from build123d import *

# Parameters (mm, degrees)
RESSALTO_EXTRUS_O1_DEPTH  = 5.25
CORTE_EXTRUS_O2_DEPTH     = 3.55
ESBO_O8_R                 = 1
CORTE_EXTRUS_O5_DEPTH     = 1.55
ESBO_O6_W                 = 1.275
ESBO_O6_H                 = 0.25
RESSALTO_EXTRUS_O2_DEPTH  = 0.025
ESBO_O7_W                 = 1.275
ESBO_O7_H                 = 0.25
CORTE_EXTRUS_O6_START     = -0.25
CORTE_EXTRUS_O6_DEPTH     = 0.25
ESBO_O10_W                = 0.445
ESBO_O10_H                = 0.25
RESSALTO_EXTRUS_O3_DEPTH  = 3.4
SIMETR_A1_COPY_1_SKETCH_W = 1.275
SIMETR_A1_COPY_1_SKETCH_H = 0.25
SIMETR_A1_COPY_1_DEPTH    = 0.025
SIMETR_A1_COPY_2_SKETCH_W = 1.275
SIMETR_A1_COPY_2_SKETCH_H = 0.25
SIMETR_A1_START           = -0.25
SIMETR_A1_COPY_3_DEPTH    = 0.25
SIMETR_A1_COPY_4_SKETCH_W = 0.445
SIMETR_A1_COPY_4_SKETCH_H = 0.25
SIMETR_A1_COPY_4_DEPTH    = 3.4


with BuildPart() as part:
    # Esboço1 → Ressalto-extrusão1 (new, symmetric)
    with BuildSketch(Plane(origin=(0, 0, 0), x_dir=(0, 0, -1), z_dir=(1, 0, 0))):
        Polygon((0.9, 3.1), (0.9, -3.1), (2.45, -3.3), (4, -3.1), (4, 3.1), (2.45, 3.3), align=None)
    extrude(amount=RESSALTO_EXTRUS_O1_DEPTH, both=True)

    # Esboço3 → Corte-extrusão2 (cut, symmetric)
    with BuildSketch(Plane(origin=(0, 0, 0), x_dir=(1, 0, 0), z_dir=(0, 1, 0))):
        Polygon((-5.25, 2.45), (-5.019897634, 4.376835982), (-6.186348907, 4.376835982), (-6.186348907, 0.523164018), (-5.019897634, 0.523164018), align=None)
    corte_extrus_o2 = extrude(amount=CORTE_EXTRUS_O2_DEPTH, both=True, mode=Mode.SUBTRACT)

    # Espelhar1: Corte-extrusão2 across plane
    add(corte_extrus_o2.mirror(Plane(origin=(0, 0, 0), x_dir=(0, 0, 1), z_dir=(1, 0, 0))), mode=Mode.SUBTRACT)

    # Esboço8 → Corte-extrusão5 (cut)
    with BuildSketch(Plane(origin=(0, 0, -4), x_dir=(-1, 0, 0), z_dir=(0, 0, -1))):
        with Locations((5.064899312, 0)):
            Circle(ESBO_O8_R)
    extrude(amount=-CORTE_EXTRUS_O5_DEPTH, mode=Mode.SUBTRACT)

    # Esboço6 → Ressalto-extrusão2 (add, symmetric)
    with BuildSketch(Plane(origin=(0, 3.3, 0), x_dir=(1, 0, 0), z_dir=(0, 1, 0))):
        with Locations((-3.8, 2.45)):
            Rectangle(ESBO_O6_W, ESBO_O6_H)
    ressalto_extrus_o2 = extrude(amount=RESSALTO_EXTRUS_O2_DEPTH, both=True)

    # Varredura1: sweep along a curve in space
    with BuildLine() as varredura1_path:
        Line((-3.8, 3.325, -2.45), (-3.8, 3.51, -2.45))
        ThreePointArc((-3.8, 3.51, -2.45), (-3.8, 3.722132034, -2.362132034), (-3.8, 3.81, -2.15))
        Line((-3.8, 3.81, -2.15), (-3.8, 3.81, 0.35))
    # Esboço7 → Varredura1 (sweep)
    with BuildSketch(Plane(origin=(0, 3.325, 0), x_dir=(1, 0, 0), z_dir=(0, 1, 0))):
        with Locations((-3.8, 2.45)):
            Rectangle(ESBO_O7_W, ESBO_O7_H)
    varredura1 = sweep(path=varredura1_path.line)

    # Esboço9 → Corte-extrusão6 (cut)
    with BuildSketch(Plane(origin=(0, 3.935, 0), x_dir=(1, 0, 0), z_dir=(0, 1, 0)).offset(CORTE_EXTRUS_O6_START)):
        Polygon((-4.0225, -0.35), (-4.4375, 0.55), (-4.4375, -0.55), (-3.1625, -0.55), (-3.1625, 0.55), (-3.5775, -0.35), align=None)
    corte_extrus_o6 = extrude(amount=CORTE_EXTRUS_O6_DEPTH, mode=Mode.SUBTRACT)

    # Esboço10 → Ressalto-extrusão3 (add)
    with BuildSketch(Plane.XY.offset(0.35)):
        with Locations((-3.8, 3.81)):
            Rectangle(ESBO_O10_W, ESBO_O10_H)
    ressalto_extrus_o3 = extrude(amount=RESSALTO_EXTRUS_O3_DEPTH)

    # Espelhar2: Ressalto-extrusão2, Varredura1, Corte-extrusão6, Ressalto-extrusão3 across plane
    add(ressalto_extrus_o2.mirror(Plane.ZX))
    add(varredura1.mirror(Plane.ZX))
    add(corte_extrus_o6.mirror(Plane.ZX), mode=Mode.SUBTRACT)
    add(ressalto_extrus_o3.mirror(Plane.ZX))

    # Simetría1: Ressalto-extrusão2, Varredura1, Corte-extrusão6, Ressalto-extrusão3 across plane
    add(ressalto_extrus_o2.mirror(Plane(origin=(0, 0, 0), x_dir=(0, 0, 1), z_dir=(1, 0, 0))))
    add(varredura1.mirror(Plane(origin=(0, 0, 0), x_dir=(0, 0, 1), z_dir=(1, 0, 0))))
    add(corte_extrus_o6.mirror(Plane(origin=(0, 0, 0), x_dir=(0, 0, 1), z_dir=(1, 0, 0))), mode=Mode.SUBTRACT)
    add(ressalto_extrus_o3.mirror(Plane(origin=(0, 0, 0), x_dir=(0, 0, 1), z_dir=(1, 0, 0))))

    # Simetría1 copy 1 sketch → Simetría1 copy 1 (add, symmetric)
    with BuildSketch(Plane(origin=(0, -3.3, 0), x_dir=(-1, 0, 0), z_dir=(0, -1, 0))):
        with Locations((-3.8, 2.45)):
            Rectangle(SIMETR_A1_COPY_1_SKETCH_W, SIMETR_A1_COPY_1_SKETCH_H)
    extrude(amount=SIMETR_A1_COPY_1_DEPTH, both=True)

    # Simetría1 copy 2: sweep along a curve in space
    with BuildLine() as simetr_a1_copy_2_path:
        Line((3.8, -3.325, -2.45), (3.8, -3.51, -2.45))
        ThreePointArc((3.8, -3.51, -2.45), (3.8, -3.722132034, -2.362132034), (3.8, -3.81, -2.15))
        Line((3.8, -3.81, -2.15), (3.8, -3.81, 0.35))
    # Simetría1 copy 2 sketch → Simetría1 copy 2 (sweep)
    with BuildSketch(Plane(origin=(0, -3.325, 0), x_dir=(-1, 0, 0), z_dir=(0, -1, 0))):
        with Locations((-3.8, 2.45)):
            Rectangle(SIMETR_A1_COPY_2_SKETCH_W, SIMETR_A1_COPY_2_SKETCH_H)
    sweep(path=simetr_a1_copy_2_path.line)

    # Simetría1 copy 3 sketch → Simetría1 copy 3 (cut)
    with BuildSketch(Plane(origin=(0, -3.935, 0), x_dir=(-1, 0, 0), z_dir=(0, -1, 0)).offset(SIMETR_A1_START)):
        Polygon((-4.0225, -0.35), (-4.4375, 0.55), (-4.4375, -0.55), (-3.1625, -0.55), (-3.1625, 0.55), (-3.5775, -0.35), align=None)
    extrude(amount=SIMETR_A1_COPY_3_DEPTH, mode=Mode.SUBTRACT)

    # Simetría1 copy 4 sketch → Simetría1 copy 4 (add)
    with BuildSketch(Plane(origin=(0, 0, 0.35), x_dir=(-1, 0, 0), z_dir=(0, 0, 1))):
        with Locations((-3.8, 3.81)):
            Rectangle(SIMETR_A1_COPY_4_SKETCH_W, SIMETR_A1_COPY_4_SKETCH_H)
    extrude(amount=SIMETR_A1_COPY_4_DEPTH)


solid = part.part
Geometry check sheet. Reference: the model listing, model coordinates, mm. A direction names the side the tool comes from. Round coordinates to 2 decimals unless told otherwise and drop trailing zeros. Order: outer loops, then holes, each group sorted by start corner. A loop starts at its lowest first (then second) coordinate and runs counter-clockwise, first axis right, second up. Notation, with made-up numbers: M -1,35.5 L 43,35.5 A27 ccw 43,54.5 Z; hole C 70,48 d8. An arc over 180 degrees is marked long. Write each question's results on one line, items separated by ' | '. Start each with the question number.
1. Set-up check for faces 1 (the face through (4, -3.935, 0)), 2 (the face through (-4, 3.685, 0)): record each of +Z, -Z, +X, -X, +Y, -Y from which the full face is reachable in a straight line by a thin tool's end or side.
2. Cross-section at D-D on x = -1.5. Record the boundary of the cut face in (y, z), plus the area to 3 significant figures.
3. Go/stop test with a flat-tipped pin: P1, Ø4, axis at x = 0, z = 2, coming from the +Y side. Record where the tip stops, or that it passes through.
4. Draft check along Y on faces 3 (the face through (-4, 3.935, 0)), 4 (the face through (-5.156, 0.046, -1.664)), 5 (the face through (-4, -3.685, 0)). Enter one of: pulls with the +Y half, pulls with the -Y half, needs draft (parallel to the pull), parting line crosses it, or undercut.
5. Cross-section at A-A on y = 0. Record the boundary of the cut face in (x, z).
6. Cross-section at C-C on z = -1.5. Give the number of separate pieces and of enclosed holes in the cut face, plus the area to 3 significant figures.
7. Cross-section at B-B on x = 3.75. Record the boundary of the cut face in (y, z) (3 decimals).
8. Material ranges on L1, parallel to Y at x = 3.75, z = 1 (3 decimals); L2, parallel to Z at x = -0.5, y = 1.5; L3, parallel to Y at x = -4, z = -1.25 (3 decimals), recorded low to high. Write a range as from..to.
Resolved:
1) face 1: +Z, -Z, +X, -X, -Y | face 2: +Z, +X, -X
2) outline: M -3.3,-2.45 L -3.1,-4 L 3.1,-4 L 3.3,-2.45 L 3.1,-0.9 L -3.1,-0.9 Z | area: 19.8 mm2
3) P1: through
4) face 3: pulls with the +Y half | face 4: needs draft | face 5: undercut
5) outline: M -5.25,-2.45 L -4.06,-2.45 L -4.06,-4 L 5.06,-4 L 5.25,-2.45 L 5.06,-0.9 L -5.06,-0.9 Z
6) separate pieces: 5 | enclosed holes: 0 | area: 66.6 mm2
7) outline: M -3.935,-2.15 A0.425 ccw -3.51,-2.575 L -3.284,-2.575 L -3.1,-4 L 3.1,-4 L 3.284,-2.575 L 3.51,-2.575 A0.425 ccw 3.935,-2.15 L 3.935,3.75 L 3.685,3.75 L 3.685,-2.15 A0.175 cw 3.51,-2.325 L 3.284,-2.325 L 3.1,-0.9 L -3.1,-0.9 L -3.284,-2.325 L -3.51,-2.325 A0.175 cw -3.685,-2.15 L -3.685,3.75 L -3.935,3.75 Z
8) L1: -3.935..-3.685, 3.685..3.935 | L2: -4..-0.9 | L3: -3.935..-3.685, -3.145..3.145, 3.685..3.935
